Check sheet for the modelled part. Datum: model origin and axes. Units: mm. Face numbers are marked on the shaded views. A direction names the side the tool comes from. Round coordinates to 2 decimals unless told otherwise and drop trailing zeros. Loops run counter-clockwise (first coordinate to the right, second up) from the corner with the lowest first, then second, coordinate; pieces in that order, holes last. Notation, with made-up numbers: (78, 39) - (89, 39) arc R15 cw to (89, 65) - close; hole circle Ø8 at (32, 68.5). An arc over 180 degrees is marked (long way). Return JSON: item names as keys, results as strings.
from build123d import *

# Parameters (mm, degrees)
F1_W           = 20.5
F1_H           = 36
F2_DEPTH       = 6
F0_W           = 16.5
F0_H           = 32
F3_DEPTH       = 4
F4_T1_DEPTH    = 68.4886593371
F5_R           = 2
F7_DEPTH       = 25
F7_DEPTH_BACK  = 20.4
F8_R           = 1
F9_W           = 10
F9_H           = 2.8
F10_DEPTH      = 25
F10_DEPTH_BACK = 25


# Not quite as in the source:
# - a fillet or chamfer that OpenCascade refuses, or shapes differently, is made with other operations: its cross-section is extruded or revolved along the edge and cut away or added


with BuildPart() as f2:
    # F1 (on Top) → F2 (new body)
    with BuildSketch(Plane.XY):
        with Locations((0.1103486419, -0.6806470305)):
            Rectangle(F1_W, F1_H)
    extrude(amount=F2_DEPTH)

    # F0 (on Top) → F3 (cut)
    with BuildSketch(Plane.XY):
        with Locations((0.1103486419, -0.6806470305)):
            Rectangle(F0_W, F0_H)
    extrude(amount=F3_DEPTH, mode=Mode.SUBTRACT)

    # F4: fillet of radius 6.5183766184 on 2 edges, made by hand

    # F4_s2 → F4_t1 (cut)
    with BuildSketch(Plane.XZ.offset(-33.5636826381)):
        with BuildLine():
            ThreePointArc((10.3603486419, 0), (8.2847350288, 4.270579832), (3.8626167745, 6))
            Line((3.8626167745, 6), (10.3603486419, 6))
            Line((10.3603486419, 6), (10.3603486419, 0))
        make_face()
        with BuildLine():
            ThreePointArc((-10.1396513581, 0), (-8.064037745, 4.270579832), (-3.6419194907, 6))
            Line((-3.6419194907, 6), (-10.1396513581, 6))
            Line((-10.1396513581, 6), (-10.1396513581, 0))
        make_face()
    extrude(amount=F4_T1_DEPTH, mode=Mode.SUBTRACT)

    # F5
    f5_edges = [f2.edges().sort_by_distance(p)[0] for p in [
        (0.110349, 17.319353, 6),
        (8.284735, 17.319353, 4.27058),
        (-8.064038, -18.680647, 4.27058),
        (-8.064038, 17.319353, 4.27058),
        (0.110349, -18.680647, 6),
        (8.284735, -18.680647, 4.27058),
    ]]
    fillet(f5_edges, radius=F5_R)

    # F6 (on Front) → F7 (cut, two sides)
    with BuildSketch(Plane.XZ) as f7_sk:
        with BuildLine():
            ThreePointArc((6.8361471832, 0), (5.8050304207, 1.791953799), (3.8626167745, 2.5))
            Line((3.8626167745, 2.5), (-3.6419194907, 2.5))
            ThreePointArc((-3.6419194907, 2.5), (-5.5843331369, 1.791953799), (-6.6154498995, 0))
            Line((-6.6154498995, 0), (6.8361471832, 0))
        make_face()
    extrude(amount=-F7_DEPTH, mode=Mode.SUBTRACT)
    extrude(f7_sk.sketch, amount=F7_DEPTH_BACK, mode=Mode.SUBTRACT)

    # F8
    f8_edges = [f2.edges().sort_by_distance(p)[0] for p in [
        (-5.584333, 15.319353, 1.791954),
        (0.110349, -16.680647, 2.5),
        (5.80503, 15.319353, 1.791954),
        (0.110349, 15.319353, 2.5),
        (5.80503, -16.680647, 1.791954),
        (-5.584333, -16.680647, 1.791954),
    ]]
    fillet(f8_edges, radius=F8_R)

    # F9 (on Right) → F10 (cut, two sides)
    with BuildSketch(Plane.YZ) as f10_sk:
        with Locations((-5, 2.2957557753)):
            Rectangle(F9_W, F9_H)
    extrude(amount=-F10_DEPTH, mode=Mode.SUBTRACT)
    extrude(f10_sk.sketch, amount=F10_DEPTH_BACK, mode=Mode.SUBTRACT)


solid = f2.part
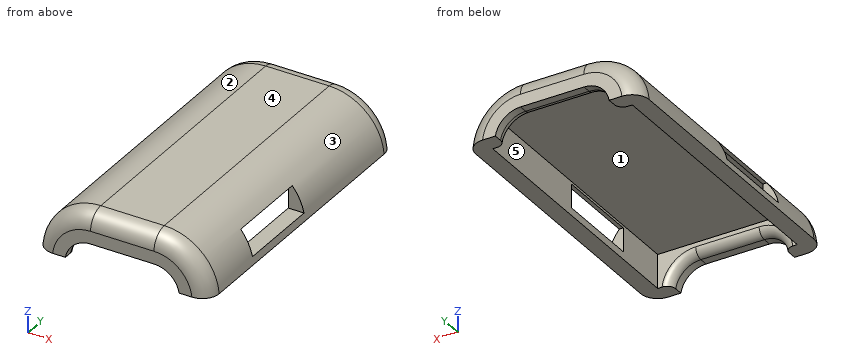
Q1. Tool access check on the marked faces 1 and 2. Record the directions out of +Z, -Z, +X, -X, +Y, -Y that give a thin tool (end or side, any length) a straight path to the whole face; none if there is none.
Answer key:
{"face 1": "-Z", "face 2": "+Z, -X, +Y, -Y"}
Q2. Depth check by flat-ended pin: P1, Ø1.5, axis at x = -0.5, y = -1, coming from the -Z side; P2, Ø0.6, axis at x = 9, z = 2, coming from the -Y side; P3, Ø0.8, axis at x = 0, y = -18.5, coming from the -Z side. Enter the tip coordinate at first touch or a pass-through.
Answer key:
{"P1": "stops at z = 4", "P2": "stops at y = -18.47", "P3": "stops at z = 2.5"}
Q3. Draft check along X on the marked faces 3, 4 and 5. Enter one of: released by +X, released by -X, zero draft, split by the parting line, or undercut.
Answer key:
{"face 3": "released by +X", "face 4": "zero draft", "face 5": "undercut"}
Q4. Sectioned sample at A-A (y = -1). Enter the section's corners in (x, z).
Answer key:
{"outline": "(-10.14, 0) - (-8.14, 0) - (-8.14, 0.9) - (-10.01, 0.9) arc R6.52 ccw to start; (-8.61, 3.7) - (-8.14, 3.7) - (-8.14, 4) - (8.36, 4) - (8.36, 3.7) - (8.84, 3.7) arc R6.52 ccw to (3.86, 6) - (-3.64, 6) arc R6.52 ccw to start; (8.36, 0) - (10.36, 0) arc R6.52 ccw to (10.23, 0.9) - (8.36, 0.9) - close"}
Q5. Sectioned sample at D-D (z = 1.5). State how many separate pieces and enclosed holes the cut face has, plus the area to 3 significant figures.
Answer key:
{"separate pieces": "4", "enclosed holes": "0", "area": "102 mm²"}
Q6. Scan lines: probe 1 along Y at (x, z) = (-7.25, 1.5); probe 2 along Z at (x, y) = (-0.5, -13.5); probe 3 along X at (y, z) = (-7, 0.75). Record each from-to range of solid material in increasing order. Write a range as [from, to].
Answer key:
{"probe 1": "y = [-18.68, -16.68], [15.32, 17.32]", "probe 2": "z = [4, 6]", "probe 3": "x = [-10.04, -8.14], [8.36, 10.26]"}
Q7. Sectioned sample at B-B (y = -13). Enter the section's corners in (x, z), plus the area to 3 significant figures.
Answer key:
{"outline": "(-10.14, 0) - (-8.14, 0) - (-8.14, 4) - (8.36, 4) - (8.36, 0) - (10.36, 0) arc R6.52 ccw to (3.86, 6) - (-3.64, 6) arc R6.52 ccw to start", "area": "39.0 mm²"}
Q8. Sectioned sample at C-C (x = -3.25). Enter the section's corners in (y, z).
Answer key:
{"outline": "(-18.68, 2.5) - (-17.68, 2.5) arc R1 ccw to (-16.68, 3.5) - (-16.68, 4) - (15.32, 4) - (15.32, 3.5) arc R1 ccw to (16.32, 2.5) - (17.32, 2.5) - (17.32, 4) arc R2 ccw to (15.32, 6) - (-16.68, 6) arc R2 ccw to (-18.68, 4) - close"}
